For this review, take the finished solid that the model builds, in its own axes (mm). Face numbers are marked on the shaded views. A direction names the side the tool comes from. Round coordinates to 2 decimals unless told otherwise and drop trailing zeros. Order: outer loops, then holes, each group sorted by start corner. A loop starts at its lowest first (then second) coordinate and runs counter-clockwise, first axis right, second up. Notation, with made-up numbers: (39, 71.25) -> (76, 71.25) arc R15 cw to (76, 89.25) -> close; hole circle Ø9 at (-25, -17). An arc over 180 degrees is marked (long way). Answer in a Markdown table with one row per item.
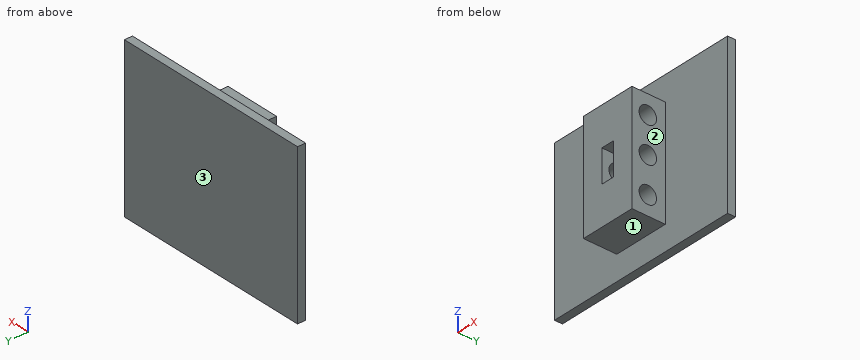
Autodesk Inventor part; units mm, degrees
ref_plane "Work Plane1" through (-21.25, 5.2, -12.9) normal (0, 0, 1) x (1, 0, 0)
ref_plane "YZ Plane" through (0, 0, 0) normal (1, 0, 0) x (0, 1, 0)
ref_plane "XZ Plane" through (0, 0, 0) normal (0, 1, 0) x (-1, 0, 0)
sketch "Sketch1" plane through (0, 0, 0) normal (0, 1, 0) x (-1, 0, 0)
  line L0 (0, 0) -> (25, 0)
  line L1 (25, 0) -> (25, -13.8)
  line L2 (25, -13.8) -> (0, -13.8)
  line L3 (0, -13.8) -> (0, 0)
  dimension "d0" = 25
  dimension "d1" = 13.8
extrude "Extrusion1" add sketch "Sketch1" along normal blind 4.2
sketch "Sketch2" plane through (0, 0, 0) normal (1, 0, 0) x (0, 0, -1)
  line L0 (0, 0) -> (0, 4.2)
  line L1 (0, 2) -> (13.8, 2)
  line L2 (13.8, 0) -> (13.8, 4.2)
  circle A0 centre (2.4, 2) radius 1.05
  circle A1 centre (11.4, 2) radius 1.05
  line L3 (0, 0) -> (13.8, 0)
  line L4 (6.9, 0) -> (6.9, 2.0025)
  line L5 (0, 4.2) -> (13.8, 4.2)
  dimension "d4" = 9
  dimension "d7" = 4.5
  dimension "d15" = 2.2
extrude "Extrusion2" cut sketch "Sketch2" against normal blind 20 contours A0 L1 | L1 A0 | A1 L1 | L1 A1
sketch "Sketch3" plane through (0, 4.2, 0) normal (0, 1, 0) x (1, 0, 0)
  line L0 (0, 6.9) -> (-25, 6.9)
  line L1 (0, -3.1) -> (-25, -3.1)
  line L2 (-25, -3.1) -> (-25, 16.9)
  line L3 (-25, 16.9) -> (0, 16.9)
  line L4 (0, 16.9) -> (0, -3.1)
  line L5 (0, -3.1) -> (-25, 16.9) construction
  line L6 (-25, -3.1) -> (0, 16.9) construction
  line L7 (-25, 13.8) -> (-25, 0)
  line L8 (0, 0) -> (0, 13.8)
  line L9 (0, 13.8) -> (-25, 13.8)
  point P0 (-12.5, 6.9)
  dimension "d10" = 20
  dimension "d11" = 6.9
  dimension "d12" = 25
extrude "Extrusion3" add sketch "Sketch3" along normal blind 1
sketch "Sketch4" plane through (0, 5.2, 0) normal (0, 1, 0) x (1, 0, 0)
  circle A0 centre (-21, 12.9) radius 0.25
  line L0 (0, 16.9) -> (-25, 16.9)
  line L1 (-25, 16.9) -> (-25, -3.1)
  line L2 (-21.25, 12.9) -> (-20.75, 12.9)
  point P0 (0, 0)
  dimension "d16" = 4
  dimension "d17" = 4
  dimension "d18" = 0.5
ref_plane "Work Plane1" through (-21.25, 5.2, -12.9) normal (0, 0, 1) x (1, 0, 0)
sketch "Sketch5" plane through (-21.25, 5.2, -12.9) normal (0, 0, 1) x (1, 0, 0)
  line L0 (-3.75, 0) -> (21.25, 0)
  line L1 (0.2469, 0) -> (0.2469, 2)
  line L2 (0.2469, 2) -> (0.9969, 0)
  line L3 (0.9969, 0) -> (0.2469, 0)
  line L4 (21.25, -1) -> (-3.75, -1)
  point P0 (21.25, -5.2)
  dimension "d21" = 2
  dimension "d28" = 0.75
revolve "Revolution1" [suppressed]
pattern_linear "Rectangular Pattern1" [suppressed]
sketch "Sketch6" plane through (0, 0, 0) normal (1, 0, 0) x (0, 0, -1)
  circle A0 centre (2.4, 2) radius 1.05
  circle A1 centre (2.4, 2) radius 1.1
  circle A2 centre (11.4, 2) radius 1.05
  circle A3 centre (11.4, 2) radius 1.1
  point P0 (0, 0)
  dimension "d29" = 2.2
  dimension "d30" = 2.2
extrude "Extrusion4" cut sketch "Sketch6" against normal blind 30.5 contours A0 | A1 | A2 | A3
sketch "Sketch7" plane through (0, 5.2, 0) normal (0, 1, 0) x (1, 0, 0)
  line L0 (0, 6.9) -> (-25, 6.9) construction
  line L1 (0, 16.9) -> (-25, 16.9)
  line L2 (-13.35, 4.85) -> (-11.65, 4.85)
  line L3 (-11.65, 4.85) -> (-11.65, 8.95)
  line L4 (-11.65, 8.95) -> (-13.35, 8.95)
  line L5 (-13.35, 8.95) -> (-13.35, 4.85)
  line L6 (-13.35, 4.85) -> (-11.65, 8.95) construction
  line L7 (-11.65, 4.85) -> (-13.35, 8.95) construction
  line L8 (0, -3.1) -> (0, 16.9)
  point P0 (0, 0)
  point P1 (-12.5, 6.9)
  dimension "d33" = 10
  dimension "d34" = 1.7
  dimension "d35" = 4.1
  dimension "d36" = 11.65
extrude "Extrusion5" cut sketch "Sketch7" against normal blind 8.45
sketch "Sketch8" plane through (0, 0, 0) normal (1, 0, 0) x (0, 0, -1)
  circle A0 centre (2.4, 2) radius 1.1
  circle A1 centre (11.4, 2) radius 1.1
  line L0 (2.4, 2) -> (11.4, 2) construction
  circle A2 centre (6.9, 2) radius 1.1
  point P0 (0, 0)
  dimension "d39" = 2.2
  dimension "d40" = 4.5
extrude "Extrusion6" cut sketch "Sketch8" against normal blind 31.95 contours A2
sketch "Sketch9" plane through (0, 5.2, 0) normal (0, 1, 0) x (1, 0, 0)
  line L0 (-13.35, 4.85) -> (-13.35, 8.95)
  line L1 (-11.65, 4.85) -> (-11.65, 8.95)
  line L2 (-13.35, 8.95) -> (-11.65, 8.95)
  line L3 (-11.65, 8.95) -> (-11.65, 4.85)
  line L4 (-11.65, 4.85) -> (-13.35, 4.85)
  line L5 (-13.35, 4.85) -> (-13.35, 8.95)
  point P0 (0, 0)
extrude "Extrusion7" add sketch "Sketch9" against normal blind 0.5
sketch "Sketch10" plane through (0, 0, 0) normal (1, 0, 0) x (0, 0, -1)
  line L0 (0, 0) -> (13.8, 0)
  line L1 (13.8, 0) -> (13.8, 4.2)
  line L2 (13.8, 4.2) -> (0, 4.2)
  line L3 (0, 4.2) -> (0, 0)
  line L4 (13.8, 4.2) -> (16.9, 4.2)
  line L5 (13.8, 0) -> (13.8, 4.2)
extrude "Extrusion8" cut sketch "Sketch10" against normal blind 9
sketch "Sketch11" plane through (-25, 0, -13.8) normal (-1, 0, 0) x (0, 0, 1)
  line L0 (13.8, 0) -> (13.8, 4.2)
  line L1 (0, 0) -> (13.8, 0)
  line L2 (13.8, 0) -> (13.8, 4.2)
  line L3 (13.8, 4.2) -> (0, 4.2)
  line L4 (0, 4.2) -> (0, 0)
  line L5 (13.8, 4.2) -> (16.9, 4.2)
extrude "Extrusion9" cut sketch "Sketch11" against normal blind 9
properties part number "Moving platform"
Q1. Take a section at D-D, the plane z = -6.9. Write out the cut boundary in (x, y), then the cut area to 4 significant figures.
Answer key:
| item | result |
|---|---|
| outline | (-25, 4.2) -> (-16, 4.2) -> (-16, 3.1) -> (-13.35, 3.1) -> (-13.35, 4.7) -> (-11.65, 4.7) -> (-11.65, 3.1) -> (-9, 3.1) -> (-9, 4.2) -> (0, 4.2) -> (0, 5.2) -> (-25, 5.2) -> close; (-16, 0) -> (-13.35, 0) -> (-13.35, 0.9) -> (-16, 0.9) -> close; (-11.65, 0) -> (-9, 0) -> (-9, 0.9) -> (-11.65, 0.9) -> close |
| area | 34.75 mm^2 |
Q2. Take a section at C-C, the plane x = -14.5. Write out the cut boundary in (y, z).
Answer key:
| item | result |
|---|---|
| outline | (0, -13.8) -> (4.2, -13.8) -> (4.2, -16.9) -> (5.2, -16.9) -> (5.2, 3.1) -> (4.2, 3.1) -> (4.2, 0) -> (0, 0) -> close; hole circle Ø2.2 at (2, -11.4); hole circle Ø2.2 at (2, -6.9); hole circle Ø2.2 at (2, -2.4) |
Q3. Tool access review of the marked faces 1, 2 and 3: name each direction out of +Z, -Z, +X, -X, +Y, -Y from which nothing blocks a thin tool from reaching the whole face with its end or side.
Answer key:
| item | result |
|---|---|
| face 1 | -Z, +X, -X, -Y |
| face 2 | +Z, -Z, +X, -Y |
| face 3 | +Z, -Z, +X, -X, +Y |
Q4. Take a section at B-B, the plane z = -11.4. Write out the cut boundary in (x, y), then the cut area to 3 significant figures.
Answer key:
| item | result |
|---|---|
| outline | (-25, 4.2) -> (-16, 4.2) -> (-16, 3.1) -> (-9, 3.1) -> (-9, 4.2) -> (0, 4.2) -> (0, 5.2) -> (-25, 5.2) -> close; (-16, 0) -> (-9, 0) -> (-9, 0.9) -> (-16, 0.9) -> close |
| area | 39.0 mm^2 |
Q5. Take a section at A-A, the plane y = 2. Write out the cut boundary in (x, z).
Answer key:
| item | result |
|---|---|
| outline | (-16, -13.8) -> (-9, -13.8) -> (-9, -12.5) -> (-16, -12.5) -> close; (-16, -10.3) -> (-9, -10.3) -> (-9, -8) -> (-11.65, -8) -> (-11.65, -8.95) -> (-13.35, -8.95) -> (-13.35, -8) -> (-16, -8) -> close; (-16, -5.8) -> (-13.35, -5.8) -> (-13.35, -4.85) -> (-11.65, -4.85) -> (-11.65, -5.8) -> (-9, -5.8) -> (-9, -3.5) -> (-16, -3.5) -> close; (-16, -1.3) -> (-9, -1.3) -> (-9, 0) -> (-16, 0) -> close |
Q6. To check wall thickness, follow probe 1 along Y at (x, z) = (-10.25, -11.4); probe 2 along Y at (x, z) = (-21.75, -6.25); probe 3 along X at (y, z) = (1.85, -1.25). State the ranges of each line that lie inside material, in increasing order.
Answer key:
| item | result |
|---|---|
| probe 1 | y = 0 to 0.9, 3.1 to 5.2 |
| probe 2 | y = 4.2 to 5.2 |
| probe 3 | x = -16 to -9 |
Q7. Clearance check with flat-ended pins moving along their axes: pin 1 Ø0.8 at (x, z) = (-12.5, -6.5) entering from -Y; pin 2 Ø2 at (y, z) = (3, -7.5) entering from -X; pin 3 Ø0.5 at (x, y) = (-12.5, 1.5) entering from +Z. State where each tip first meets the part, or that it passes through.
Answer key:
| item | result |
|---|---|
| pin 1 | stops at y = 4.7 |
| pin 2 | stops at x = -16 |
| pin 3 | stops at z = 0 |
